Check sheet for the modelled part. Datum: model origin and axes. Units: mm. A direction names the side the tool comes from. Coordinates: 2 decimals unless noted, no trailing zeros. Order: outer loops, then holes, each group sorted by start corner. A loop starts at its lowest first (then second) coordinate and runs counter-clockwise, first axis right, second up. Notation, with made-up numbers: (-28, 0) -> (-5, 0) arc R7 ccw to (-5, 9) -> close; hole circle Ø11 at (51.25, 58.25). An arc over 180 degrees is marked (long way). Put each result on its own line as item: value. Start each with the question number.
```python
from build123d import *

# Parameters (mm, degrees)
SKETCH_1_R          = 4.5
EXTRUDE_1_DEPTH     = 35
SKETCH_2_W          = 6
SKETCH_2_H          = 6.708203932
EXTRUDE_2_DEPTH     = 9
SKETCH_3_R          = 2
CUT_EXTRUDE_1_DEPTH = 45.860896112
FILLET_1_R          = 1


with BuildPart() as part:
    # Эскиз1 → Бобышка-Вытянуть1 (new body)
    with BuildSketch(Plane.XY):
        Circle(SKETCH_1_R)
    extrude(amount=EXTRUDE_1_DEPTH)

    # Эскиз2 → Бобышка-Вытянуть2 (add)
    with BuildSketch(Plane.XY.offset(35)):
        with BuildLine():
            Line((-3, 3.354101966), (3, 3.354101966))
            ThreePointArc((3, 3.354101966), (0, 4.5), (-3, 3.354101966))
        make_face()
        Rectangle(SKETCH_2_W, SKETCH_2_H)
        with BuildLine():
            ThreePointArc((-3, -3.354101966), (0, -4.5), (3, -3.354101966))
            Line((3, -3.354101966), (-3, -3.354101966))
        make_face()
    extrude(amount=EXTRUDE_2_DEPTH)

    # Эскиз3 → Вырез-Вытянуть1 (cut, through all)
    with BuildSketch(Plane.ZY.offset(3)):
        with Locations((39.7, 0)):
            Circle(SKETCH_3_R)
    extrude(amount=-CUT_EXTRUDE_1_DEPTH, mode=Mode.SUBTRACT)

    # Скругление1
    fillet_1_edges = [part.edges().sort_by_distance(p)[0] for p in [
        (0, 4.5, 44),
        (0, -4.5, 44),
    ]]
    fillet(fillet_1_edges, radius=FILLET_1_R)


solid = part.part
```
1) Scan lines: line 1 along Y through (x, z) = (-0.95, 39.7); line 2 along Y through (x, z) = (0.5, 39.7); line 3 along Y through (x, z) = (3, 4). Record each from-to range of solid material in increasing order. Write a range as [from, to].
2) Sectioned sample at A-A (y = 0). Record the boundary of the cut face in (x, z), plus the area to 3 significant figures.
3) Sectioned sample at B-B (z = 39.7). Record the boundary of the cut face in (x, y), plus the area to 3 significant figures.
4) Sectioned sample at C-C (x = 0). Record the boundary of the cut face in (y, z), plus the area to 3 significant figures.
5) Gauge pin test, flat ends, axial feed: pin 1 (2 mm diameter, centred on y = -1, z = 38.5, fed in from -X); pin 2 (2 mm diameter, centred on x = -1.5, z = 15.5, fed in from +Y); pin 3 (3 mm diameter, centred on x = -2.5, z = 37.5, fed in from +Y). Record the tip position at first contact, or that the pin passes through.
6) Sectioned sample at D-D (z = 21). Record the boundary of the cut face in (x, y), plus the area to 3 significant figures.
7) Access from +Z, -Z, +X, -X, +Y, -Y to the whole of each face (thin tool, end or side, straight path). Record for faces 1 (the flat face through (-4, 0, 35)), 2 (the flat face through (3, 0, 37)), 3 (the flat face through (0, 0, 44)).
Entries:
1. line 1: y = [-4.4, -2], [2, 4.4]
1. line 2: y = [-4.47, -2], [2, 4.47]
1. line 3: y = [-3.35, 3.35]
2. outline: (-4.5, 0) -> (4.5, 0) -> (4.5, 35) -> (3, 35) -> (3, 37.7) -> (-3, 37.7) -> (-3, 35) -> (-4.5, 35) -> close; (-3, 41.7) -> (3, 41.7) -> (3, 44) -> (-3, 44) -> close
2. area: 345 mm2
3. outline: (-3, -3.35) arc R4.5 ccw to (3, -3.35) -> (3, -2) -> (-3, -2) -> close; (-3, 2) -> (3, 2) -> (3, 3.35) arc R4.5 ccw to (-3, 3.35) -> close
3. area: 25.7 mm2
4. outline: (-4.5, 0) -> (4.5, 0) -> (4.5, 43) arc R1 ccw to (3.5, 44) -> (-3.5, 44) arc R1 ccw to (-4.5, 43) -> close; hole circle Ø4 at (0, 39.7)
4. area: 383 mm2
5. pin 1: stops at x = -3
5. pin 2: stops at y = 4.47
5. pin 3: stops at y = 4.39
6. outline: circle Ø9 at (0, 0)
6. area: 63.6 mm2
7. face 1: +Z, -X, +Y, -Y
7. face 2: +Z, +X, +Y, -Y
7. face 3: +Z, +X, -X, +Y, -Y
